from build123d import *

# Parameters (mm, degrees)
SKETCH_1_W          = 20
SKETCH_1_H          = 4
CHAMFER_1_SIZE      = 1.35
SKETCH_2_W          = 3.34427191
SKETCH_2_H          = 1.2
CUT_EXTRUDE_1_DEPTH = 5


with BuildPart() as part:
    # Эскиз1 → Повернуть1 (revolve)
    with BuildSketch(Plane(origin=(0, 0, 0), x_dir=(0, 0, -1), z_dir=(1, 0, 0))):
        with BuildLine():
            Line((-10, 0), (-10, 4))
            ThreePointArc((-10, 4), (-11.132898199, 2.140932539), (-11.527864045, 0))
            Line((-11.527864045, 0), (-10, 0))
        make_face()
        with Locations((0, 2)):
            Rectangle(SKETCH_1_W, SKETCH_1_H)
    revolve(axis=Axis((0, 0, -10), (0, 0, 1)))

    # Фаска1
    chamfer_1_edges = [part.edges().sort_by_distance(p)[0] for p in [
        (0, -4, -10),
    ]]
    chamfer(chamfer_1_edges, length=CHAMFER_1_SIZE)

    # Эскиз2 → Вырез-Вытянуть1 (cut, symmetric)
    with BuildSketch(Plane(origin=(0, 0, 0), x_dir=(0, 0, -1), z_dir=(1, 0, 0))):
        with Locations((-10, 0)):
            Rectangle(SKETCH_2_W, SKETCH_2_H)
    extrude(amount=CUT_EXTRUDE_1_DEPTH, both=True, mode=Mode.SUBTRACT)


solid = part.part
Read the model definition and answer for the solid it produces. Units are mm, in the model's axes. Coordinates: 2 decimals unless noted, no trailing zeros. Loops run counter-clockwise (first coordinate to the right, second up) from the corner with the lowest first, then second, coordinate; pieces in that order, holes last.
Q1. The part is cut by section D-D on z = -7. Write down the section's boundary in (x, y).
Q2. The part is cut by section A-A on z = 8.75. Write down the section's boundary in (x, y), and give its area (3 significant figures).
Q3. The part is cut by section C-C on y = 0. Write down the section's boundary in (x, z).
Q4. The mould has two halves that part along Y. Classify faces 1 (the face through (0, 0, -10)), 2 (the face through (3.905, -0.867, 0.544)), 3 (the face through (0, 0, 8.328)): +Y half, -Y half, draft (parallel to the pull), parting line (faces both ways), or undercut.
Q5. The part is cut by section B-B on x = 0. Write down the section's boundary in (y, z).
Q6. Consider probe 1 along Z at (x, y) = (1.5, 0); probe 2 along Z at (x, y) = (-2.25, 0.75); probe 3 along X at (y, z) = (-2.5, 4.5). Determine where each line is inside the solid, lowest interval first.
Q7. Each of these flat-tipped pins is pushed along its axis until it touches: pin 1 Ø1.5 at (y, z) = (1.5, -3) entering from -X; pin 2 Ø1 at (x, z) = (-1.5, 9.5) entering from +Y. Where does it stop, or does it pass through?
Results below:
1. outline: circle Ø8 at (0, 0)
2. outline: (-3.95, -0.6) arc R4 ccw to (3.95, -0.6) - close; (-3.95, 0.6) - (3.95, 0.6) arc R4 ccw to start
2. area: 40.7 mm2
3. outline: (-4, -8.65) - (-2.65, -10) - (2.65, -10) - (4, -8.65) - (4, 8.33) - (-4, 8.33) - close
4. face 1: draft
4. face 2: parting line
4. face 3: undercut
5. outline: (-4, -8.65) - (-2.65, -10) - (2.65, -10) - (4, -8.65) - (4, 10) arc R6 ccw to (0.6, 11.5) - (0.6, 8.33) - (-0.6, 8.33) - (-0.6, 11.5) arc R6 ccw to (-4, 10) - close
6. probe 1: z = -10 to 8.33
6. probe 2: z = -10 to 11.04
6. probe 3: x = -3.12 to 3.12
7. pin 1: stops at x = -3.93
7. pin 2: stops at y = 3.87
